Read the model definition and answer for the solid it produces. Units are mm, in the model's axes. A direction names the side the tool comes from. Coordinates: 2 decimals unless noted, no trailing zeros. Loops run counter-clockwise (first coordinate to the right, second up) from the corner with the lowest first, then second, coordinate; pieces in that order, holes last.
Q1. Section D-D (y = 2.5) is taken. Give the vertices of the cut face in (x, z) (3 decimals).
Q2. Section A-A (x = 15.24) is taken. Give the vertices of the cut face in (y, z) (3 decimals).
Q3. Section C-C (x = 79.5) is taken. Give the vertices of the cut face in (y, z) (3 decimals).
Q4. The mould has two halves that part along X. Classify faces 3 (the face through (0, 23, 8)), 4 (the face through (66, 13, 0)), 5 (the face through (114.704, 9.963, 1.565)): pulls with the +X half, pulls with the -X half, needs draft (parallel to the pull), parting line crosses it, or undercut.
Q5. Which of the six approach directions +Z, -Z, +X, -X, +Y, -Y give full straight-line access (tool end or side, diameter ignored) to faces 1 (the face through (66, 11, 3.175)), 2 (the face through (103, 24, 25.4))?
Q6. Section B-B (y = 8.89) is taken. Give the vertices of the cut face in (x, z) (3 decimals), then the cut area to 3 significant figures.
Q7. Straight lines are drawn through the part: line 1 (Y direction, x = 118.11, z = 2.45); line 2 (Z direction, x = 18, y = 19.75) (3 decimals); line 3 (Y direction, x = 79, z = 20) (3 decimals). For each, find the intervals that lie inside material, in ascending order.
Q8. Flat-ended cylindrical pins translate along their axes: P1, Ø5.5, axis at x = 15.24, y = 8.89, coming from the +Z side; P2, Ø1, axis at x = 46, z = 10.5, coming from the -Y side (3 decimals). Find the tip coordinate at first contact, or state that the pin passes through.
from build123d import *

# Parameters (mm, degrees)
BOSS_EXTRUDE1_DEPTH = 133.35
SKETCH5_R           = 3.57124
CUT_EXTRUDE1_DEPTH  = 139.103376269


with BuildPart() as part:
    # Sketch1 → Boss-Extrude1 (new body)
    with BuildSketch(Plane(origin=(0, 0, 0), x_dir=(0, 0, -1), z_dir=(1, 0, 0))):
        Polygon((0, 0), (0, 25.4), (-25.4, 25.4), (-25.4, 22.225), (-3.175, 22.225), (-3.175, 0), align=None)
    extrude(amount=BOSS_EXTRUDE1_DEPTH)

    # Cut-Sweep1: read off the stored shape, not the designer's step
    # Cut-Sweep1: loft between two sections, ruled curve by curve
    cut_sweep1_from = [
        Edge.make_bspline([(317.515141944, -384.873460742, 110.314894304), (318.529967826, -386.50832307, 135.641902686), (340.110332702, -373.112508356, 135.641902686), (339.095506819, -371.477646028, 110.314894304), (338.080680937, -369.8427837, 84.987885922), (316.500316061, -383.238598413, 84.987885922), (317.515141944, -384.873460742, 110.314894304)], [0, 0, 0, 0, 0.5, 0.5, 0.5, 1, 1, 1, 1], 3, [1, 0.333333333, 0.333333333, 1, 0.333333333, 0.333333333, 1]),
    ]
    cut_sweep1_to = [
        Edge.make_bspline([(-268.15000351, 494.008408115, -89.503953221), (-267.135177627, 492.373545787, -64.176944839), (-245.554812752, 505.769360501, -64.176944839), (-246.569638634, 507.404222829, -89.503953221), (-247.584464517, 509.039085157, -114.830961603), (-269.164829392, 495.643270444, -114.830961603), (-268.15000351, 494.008408115, -89.503953221)], [0, 0, 0, 0, 0.5, 0.5, 0.5, 1, 1, 1, 1], 3, [1, 0.333333333, 0.333333333, 1, 0.333333333, 0.333333333, 1]),
    ]
    cut_sweep1 = Solid(Shell([*[Face.make_surface_from_curves(cut_sweep1_from[k], cut_sweep1_to[k]) for k in range(1)], Face(Wire(cut_sweep1_from)), Face(Wire(cut_sweep1_to))]))
    add(cut_sweep1, mode=Mode.SUBTRACT)

    # Sketch5 → Cut-Extrude1 (cut, through all)
    with BuildSketch(Plane(origin=(0, 0, 0), x_dir=(-1, 0, 0), z_dir=(0, 0, -1))):
        with Locations((-118.11, 8.89)):
            Circle(SKETCH5_R)
        with Locations((-15.24, 8.89)):
            Circle(SKETCH5_R)
    extrude(amount=-CUT_EXTRUDE1_DEPTH, mode=Mode.SUBTRACT)


solid = part.part
Numbers:
1. outline: (0, 0) - (133.35, 0) - (133.35, 3.175) - (0, 3.175) - close
2. outline: (0, 0) - (5.319, 0) - (5.319, 3.175) - (0, 3.175) - close; (12.461, 0) - (25.4, 0) - (25.4, 25.4) - (22.225, 25.4) - (22.225, 3.175) - (12.461, 3.175) - close
3. outline: (0, 0) - (25.4, 0) - (25.4, 25.4) - (22.225, 25.4) - (22.225, 3.175) - (0, 3.175) - close
4. face 3: pulls with the -X half
4. face 4: needs draft
4. face 5: undercut
5. face 1: +Z, +X, -X, -Y
5. face 2: +Z, +X, -X, +Y, -Y
6. outline: (0, 0) - (11.669, 0) - (11.669, 3.175) - (0, 3.175) - close; (18.811, 0) - (114.539, 0) - (114.539, 3.175) - (18.811, 3.175) - close; (121.681, 0) - (133.35, 0) - (133.35, 3.175) - (121.681, 3.175) - close
6. area: 378 mm2
7. line 1: y = 0 to 5.32, 12.46 to 25.4
7. line 2: z = 0 to 3.175
7. line 3: y = 22.225 to 25.4
8. P1: passes through
8. P2: stops at y = 22.225
